Input: part model. Units: mm. Frame: model coordinates. Face numbers are marked on the shaded views. A direction names the side the tool comes from. Coordinates: 2 decimals unless noted, no trailing zeros. Write each loop counter-clockwise with the first axis right and the second up, starting at its lowest first coordinate (ties: lowest second). Pieces come first, ordered by that corner, then holes. Notation, with made-up numbers: (27.25, 61) - (69.25, 61) arc R18 cw to (69.25, 82) - close; hole circle Ø1 at (44.5, -35). An arc over 180 degrees is marked (long way). Put each result on its own line as item: value. Start each with the question number.
1. Access query for the marked faces 1 and 2. Directions: +Z, -Z, +X, -X, +Y, -Y. A direction counts if a zero-diameter tool reaches every point of the face in a straight line with its end or side. Return the directions, or none.
2. Line query: line 1 (Z direction, x = 28, y = 14.5); line 2 (X direction, y = 17, z = 27); line 3 (X direction, y = 12.75, z = 27.5). Output: solid intervals per line, ascending.
3. Cut plane B-B, the plane y = 16.5. Return loops of the section in (x, z).
4. Pin query (flat end, axial travel): pin 1 (7 mm diameter, centred on x = 28, z = 20.5, fed in from +Y); pin 2 (2.5 mm diameter, centred on x = 30, z = 12, fed in from +Y). Return the tip coordinate at first contact, or that it passes through.
5. Cut plane C-C, the plane x = 63. Return loops of the section in (y, z).
6. Cut plane A-A, the plane z = 20. Return loops of the section in (x, y).
from build123d import *

# Parameters (mm, degrees)
SALIENTE_EXTRUIR1_DEPTH = 34.5
CROQUIS2_R              = 9
CORTAR_EXTRUIR1_DEPTH   = 26
CROQUIS3_W              = 10
CROQUIS3_H              = 5
CROQUIS3_W_2            = 10.5
CROQUIS3_W_3            = 20.5
CORTAR_EXTRUIR2_DEPTH   = 3.5


with BuildPart() as part:
    # Croquis1 → Saliente-Extruir1 (new body)
    with BuildSketch(Plane.XY):
        Polygon((0, 0), (0, 18), (16.5, 18), (16.5, 15), (39, 15), (39, 18), (87, 18), (87, 15), (109.5, 15), (109.5, 18), (126, 18), (126, 0), align=None)
    extrude(amount=SALIENTE_EXTRUIR1_DEPTH)

    # Croquis2 → Cortar-Extruir1 (cut)
    with BuildSketch(Plane(origin=(0, 0, 0), x_dir=(-1, 0, 0), z_dir=(0, 0, -1))):
        with Locations((-63, 18)):
            Circle(CROQUIS2_R)
    extrude(amount=-CORTAR_EXTRUIR1_DEPTH, mode=Mode.SUBTRACT)

    # Croquis3 → Cortar-Extruir2 (cut)
    with BuildSketch(Plane(origin=(0, 15, 0), x_dir=(1, 0, 0), z_dir=(0, 1, 0))):
        with Locations((22.5, -29)):
            Rectangle(CROQUIS3_W, CROQUIS3_H)
        with Locations((32.75, -29)):
            Rectangle(CROQUIS3_W_2, CROQUIS3_H)
        with Locations((32.75, -21)):
            Rectangle(CROQUIS3_W_2, CROQUIS3_H)
        with Locations((22.5, -21)):
            Rectangle(CROQUIS3_W, CROQUIS3_H)
        with Locations((32.75, -13)):
            Rectangle(CROQUIS3_W_2, CROQUIS3_H)
        with Locations((22.5, -13)):
            Rectangle(CROQUIS3_W, CROQUIS3_H)
        with Locations((32.75, -5)):
            Rectangle(CROQUIS3_W_2, CROQUIS3_H)
        with Locations((22.5, -5)):
            Rectangle(CROQUIS3_W, CROQUIS3_H)
        with Locations((98.25, -29)):
            Rectangle(CROQUIS3_W_3, CROQUIS3_H)
        with Locations((98.25, -21)):
            Rectangle(CROQUIS3_W_3, CROQUIS3_H)
        with Locations((98.25, -13)):
            Rectangle(CROQUIS3_W_3, CROQUIS3_H)
        with Locations((98.25, -5)):
            Rectangle(CROQUIS3_W_3, CROQUIS3_H)
    extrude(amount=-CORTAR_EXTRUIR2_DEPTH, mode=Mode.SUBTRACT)


solid = part.part
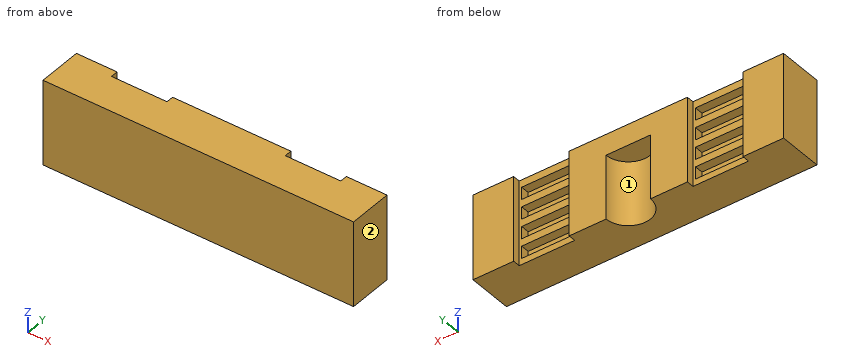
Report:
1. face 1: -Z, +Y
1. face 2: +Z, -Z, +X, +Y, -Y
2. line 1: z = 0 to 2.5, 7.5 to 10.5, 15.5 to 18.5, 23.5 to 26.5, 31.5 to 34.5
2. line 2: x = 0 to 16.5, 39 to 87, 109.5 to 126
2. line 3: x = 0 to 17.5, 38 to 88, 108.5 to 126
3. outline: (0, 0) - (16.5, 0) - (16.5, 34.5) - (0, 34.5) - close; (39, 0) - (54.13, 0) - (54.13, 26) - (71.87, 26) - (71.87, 0) - (87, 0) - (87, 34.5) - (39, 34.5) - close; (109.5, 0) - (126, 0) - (126, 34.5) - (109.5, 34.5) - close
4. pin 1: stops at y = 15
4. pin 2: stops at y = 11.5
5. outline: (0, 0) - (9, 0) - (9, 26) - (18, 26) - (18, 34.5) - (0, 34.5) - close
6. outline: (0, 0) - (126, 0) - (126, 18) - (109.5, 18) - (109.5, 15) - (108.5, 15) - (108.5, 11.5) - (88, 11.5) - (88, 15) - (87, 15) - (87, 18) - (72, 18) arc R9 cw to (54, 18) - (39, 18) - (39, 15) - (38, 15) - (38, 11.5) - (17.5, 11.5) - (17.5, 15) - (16.5, 15) - (16.5, 18) - (0, 18) - close
